CAD build for the part. Positions are in the model's coordinates, mm. Coordinates: 2 decimals unless noted, no trailing zeros. Order: outer loops, then holes, each group sorted by start corner. A loop starts at its lowest first (then second) coordinate and runs counter-clockwise, first axis right, second up. Notation, with made-up numbers: M 45,32.25 L 64,32.25 A17 ccw 64,42.25 Z; hole C 76,-3 d7. An arc over 180 degrees is marked long. Write item = value, one per line.
from build123d import *

# Parameters (mm, degrees)
F1_DEPTH = 3


with BuildPart() as f1:
    # F0 (on Top) → F1 (new body)
    with BuildSketch(Plane.XY):
        with BuildLine():
            Line((2.170431, -46.027672), (-41.079569, -46.027672))
            ThreePointArc((-41.079569, -46.027672), (-27.642472, -66.108974), (-5.829569, -76.501831))
            ThreePointArc((-5.829569, -76.501831), (-1.845179, -77.032088), (2.170431, -77.209299))
            Line((2.170431, -77.209299), (2.170431, -46.027672))
        make_face()
        with BuildLine():
            ThreePointArc((10.170431, -76.501831), (31.983335, -66.108974), (45.420431, -46.027672))
            Line((45.420431, -46.027672), (2.170431, -46.027672))
            Line((2.170431, -46.027672), (2.170431, -77.209299))
            ThreePointArc((2.170431, -77.209299), (6.186042, -77.032088), (10.170431, -76.501831))
        make_face()
        Polygon((45.420431, 29.972328), (-41.079569, 29.972328), (-41.079569, -46.027672), (2.170431, -46.027672), (45.420431, -46.027672), align=None)
        with BuildLine():
            ThreePointArc((2.170431, -77.209299), (-1.845179, -77.032088), (-5.829569, -76.501831))
            Line((-5.829569, -76.501831), (-5.829569, -78.805961))
            Line((-5.829569, -78.805961), (2.170431, -78.805961))
            Line((2.170431, -78.805961), (10.170431, -78.805961))
            Line((10.170431, -78.805961), (10.170431, -76.501831))
            ThreePointArc((10.170431, -76.501831), (6.186042, -77.032088), (2.170431, -77.209299))
        make_face()
    extrude(amount=F1_DEPTH)


solid = f1.part
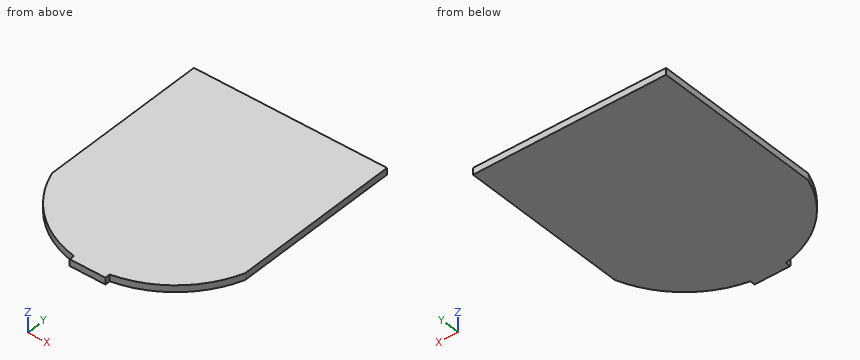
(1) Slice it at B-B, the plane x = -19. Write the cut outline in (y, z), then the cut area to 3 significant figures.
Evaluation:
outline = M -72,0 L 29.97,0 L 29.97,3 L -72,3 Z
area = 306 mm²
(2) Slice it at A-A, the plane z = 1.4. Write the cut outline in (x, y), then the cut area to 3 significant figures.
Evaluation:
outline = M -41.08,-46.03 A45.59 ccw -5.83,-76.5 L -5.83,-78.81 L 10.17,-78.81 L 10.17,-76.5 A45.59 ccw 45.42,-46.03 L 45.42,29.97 L -41.08,29.97 Z
area = 8,580 mm²
(3) Wall check: line 1 (Y direction, x = 37, z = 2.2); line 2 (Y direction, x = 20.5, z = 0.35); line 3 (X direction, y = -58, z = 1.5). Give the ranges that are in metal, low to high. Write a range as from..to.
Evaluation:
line_1 = -61.03..29.97
line_2 = -73.36..29.97
line_3 = -35.01..39.35
(4) Slice it at C-C, the plane y = -60.5. Write the cut outline in (x, z), then the cut area to 3 significant figures.
Evaluation:
outline = M -33.1,0 L 37.44,0 L 37.44,3 L -33.1,3 Z
area = 212 mm²
